Autodesk Inventor part; units mm, degrees
ref_plane "YZ Plane" through (0, 0, 0) normal (1, 0, 0) x (0, 1, 0)
ref_plane "XZ Plane" through (0, 0, 0) normal (0, 1, 0) x (-1, 0, 0)
ref_plane "XY Plane" through (0, 0, 0) normal (0, 0, 1) x (1, 0, 0)
sketch "Sketch1" plane through (0, 0, 0) normal (0, 0, 1) x (1, 0, 0)
  circle A0 centre (0, 0) radius 16
  dimension "d0" = 32
extrude "Extrusion1" add sketch "Sketch1" along normal blind 10
sketch "Sketch3" plane through (0, 0, 0) normal (0, 0, -1) x (-1, 0, 0)
  circle A0 centre (0, 0) radius 10
  dimension "d9" = 20
extrude "Extrusion3" add sketch "Sketch3" along normal blind 3
sketch "Sketch2" plane through (0, 0, 10) normal (0, 0, 1) x (1, 0, 0)
  circle A0 centre (-4, 0) radius 2.1
  circle A1 centre (4, 0) radius 2.1
  point P0 (0, 0)
  dimension "d3" = 4
  dimension "d4" = 4
  dimension "d5" = 4.2
  dimension "d6" = 4.2
extrude "Extrusion2" cut sketch "Sketch2" against normal through all
properties part number "Remskive to huller"
Can you work these out from the model? Positions are in its coordinate system, mm. A direction names the side the tool comes from. Give positions to 0.01 mm unless a question says otherwise; leave off trailing zeros. Order: outer loops, then holes, each group sorted by start corner. A loop starts at its lowest first (then second) coordinate and runs counter-clockwise, first axis right, second up. Notation, with made-up numbers: M -26.75,51 L 7.25,51 A25 ccw 7.25,79 Z; hole C 40.5,43.5 d6. An arc over 180 degrees is marked long. Write item = value, one per line. Start each with the question number.
Q1. Suppose I cut it at A-A (y = 0). Write out the boundary of the cut face in (x, z).
Q2. For faces 1 (the flat face through (-0.2, -10.4, 0)), 2 (the cylindrical face through (-6.1, 0.09, 3.59)), which set-ups out of +Z, -Z, +X, -X, +Y, -Y let a thin tool reach every point of the face, with its end or its side?
Q3. Suppose I cut it at B-B (x = 4). Write out the boundary of the cut face in (y, z), plus the area to 3 significant figures.
Q4. Suppose I cut it at D-D (x = 0). Write out the boundary of the cut face in (y, z).
Q5. I need wall thicknesses on probe 1 along Y at (x, z) = (-5, 2.5); probe 2 along Z at (x, y) = (-13, -8); probe 3 along X at (y, z) = (-0.5, 7.25). Which ranges of each line are inside material? Lowest first, please. Write a range as [from, to].
Q6. Suppose I cut it at C-C (z = 6.25). Write out the boundary of the cut face in (x, y), plus the area to 3 significant figures.
Q7. We'd pull the mould along Y, two halves only. Please class faces 3 (the flat face through (0, 0, -3)), 4 (the cylindrical face through (-3.47, 15.62, 4.93)), 5 (the cylindrical face through (6.003, 0.631, 3.591)): pulls with the +Y half, pulls with the -Y half, needs draft (parallel to the pull), parting line crosses it, or undercut.
Q8. Will these pins go through, and if not, where does the flat tip stop? pin 1 Ø5 at (x, z) = (7.5, 3) entering from -Y; pin 2 Ø2 at (x, z) = (-5.5, 1) entering from +Y; pin 3 Ø3 at (x, z) = (9, 7) entering from +Y.
Check result:
q1.outline = M -16,0 L -10,0 L -10,-3 L -6.1,-3 L -6.1,10 L -16,10 Z; M -1.9,-3 L 1.9,-3 L 1.9,10 L -1.9,10 Z; M 6.1,-3 L 10,-3 L 10,0 L 16,0 L 16,10 L 6.1,10 Z
q2.face_1 = -Z
q2.face_2 = +Z, -Z
q3.outline = M -15.49,0 L -9.17,0 L -9.17,-3 L -2.1,-3 L -2.1,10 L -15.49,10 Z; M 2.1,-3 L 9.17,-3 L 9.17,0 L 15.49,0 L 15.49,10 L 2.1,10 Z
q3.area = 310 mm2
q4.outline = M -16,0 L -10,0 L -10,-3 L 10,-3 L 10,0 L 16,0 L 16,10 L -16,10 Z
q5.probe_1 = [-15.2, -1.85], [1.85, 15.2]
q5.probe_2 = [0, 10]
q5.probe_3 = [-15.99, -6.04], [-1.96, 1.96], [6.04, 15.99]
q6.outline = C 0,0 d32; hole C -4,0 d4.2; hole C 4,0 d4.2
q6.area = 777 mm2
q7.face_3 = needs draft
q7.face_4 = parting line crosses it
q7.face_5 = undercut
q8.pin_1 = -15.2
q8.pin_2 = 15.35
q8.pin_3 = 14.13
